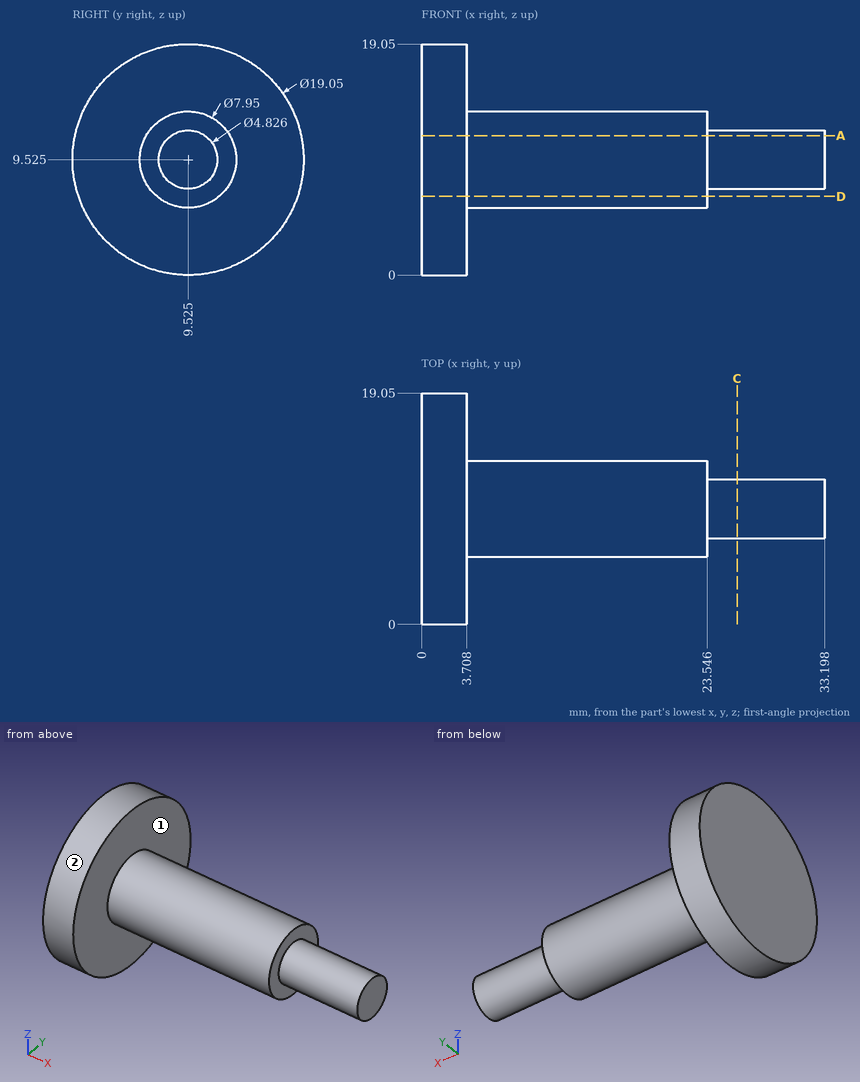
Here's the drawing with two shaded views (mm, measured from the low corner). I have some questions. A direction names the side the tool comes from. Give positions to 0.01 mm unless a question says otherwise; leave off trailing zeros. Order: outer loops, then holes, each group sorted by start corner. A loop starts at its lowest first (then second) coordinate and runs counter-clockwise, first axis right, second up. Notation, with made-up numbers: (2.25, 57.5) - (11.25, 57.5) arc R19 cw to (11.25, 61.5) - close; hole circle Ø9 at (-6.75, 8). An arc over 180 degrees is marked (long way). Write each question's results on one line, items separated by ' | '.
1) Suppose I cut it at A-A, the plane z = 11.5. Write out the boundary of the cut face in (x, y) (1 decimal).
Final values:
outline: (0, 0.2) - (3.7, 0.2) - (3.7, 6.1) - (23.5, 6.1) - (23.5, 8.1) - (33.2, 8.1) - (33.2, 10.9) - (23.5, 10.9) - (23.5, 13) - (3.7, 13) - (3.7, 18.8) - (0, 18.8) - close
2) Suppose I cut it at D-D, the plane z = 6.5. Write out the boundary of the cut face in (x, y) (1 decimal).
Final values:
outline: (0, 0.5) - (3.7, 0.5) - (3.7, 6.9) - (23.5, 6.9) - (23.5, 12.1) - (3.7, 12.1) - (3.7, 18.6) - (0, 18.6) - close
3) Suppose I cut it at C-C, the plane x = 26. Write out the boundary of the cut face in (y, z) (1 decimal).
Final values:
outline: circle Ø4.8 at (9.5, 9.5)
4) Please list where these lines run through material, in increasing order: line 1 along X through (y, z) = (4.75, 13); line 2 along Y through (x, z) = (12, 9.5); line 3 along Z through (x, y) = (22.5, 6.75). Write a range as [from, to].
Final values:
line 1: x = [0, 3.71] | line 2: y = [5.55, 13.5] | line 3: z = [6.68, 12.37]
5) On a 3-axis mill with a long thin cutter (end or side, diameter ignored), from which of +Z, -Z, +X, -X, +Y, -Y can I reach the whole of each face in a straight line? I mean the marked faces 1 and 2. Say none if no direction works.
Final values:
face 1: +X | face 2: +X, -X
6) I'm going to push flat-ended pins straight in: pin 1 Ø3 at (x, z) = (18.5, 14.5) entering from +Y (1 decimal); pin 2 Ø8 at (x, y) = (14, 2.5) entering from +Z (1 decimal); pin 3 Ø8 at (x, y) = (29.5, 10) entering from -Z; pin 4 Ø2 at (x, z) = (28, 14.5) entering from +Y. Where does each tip first touch, or does it pass through?
Final values:
pin 1: stops at y = 11.5 | pin 2: stops at z = 12.1 | pin 3: stops at z = 7.11 | pin 4: passes through
